Input: part model. Units: mm. Frame: model coordinates. A direction names the side the tool comes from. Coordinates: 2 decimals unless noted, no trailing zeros. Loops run counter-clockwise (first coordinate to the right, second up) from the corner with the lowest first, then second, coordinate; pieces in that order, holes last. Notation, with made-up numbers: (86.5, 65) - (111.5, 65) arc R9 cw to (111.5, 72) - close; hole circle Ø5 at (56, 72.25). An arc over 180 degrees is marked (long way). Use one line per item in the form item = value.
from build123d import *

# Parameters (mm, degrees)
CROQUIS1_W              = 93
CROQUIS1_H              = 56
SALIENTE_EXTRUIR1_DEPTH = 2.6
CROQUIS2_W              = 10
CROQUIS2_H              = 2.5
CORTAR_EXTRUIR1_DEPTH   = 2.6
CROQUIS3_W              = 6
CROQUIS3_H              = 1.5
CROQUIS3_H_2            = 3
SALIENTE_EXTRUIR2_DEPTH = 2.6


with BuildPart() as part:
    # Croquis1 → Saliente-Extruir1 (new body)
    with BuildSketch(Plane(origin=(0, 0, 0), x_dir=(1, 0, 0), z_dir=(0, 1, 0))):
        Rectangle(CROQUIS1_W, CROQUIS1_H)
    extrude(amount=SALIENTE_EXTRUIR1_DEPTH)

    # Croquis2 → Cortar-Extruir1 (cut)
    with BuildSketch(Plane(origin=(0, 2.6, 0), x_dir=(1, 0, 0), z_dir=(0, 1, 0))):
        with Locations((0, 26.75)):
            Rectangle(CROQUIS2_W, CROQUIS2_H)
    extrude(amount=-CORTAR_EXTRUIR1_DEPTH, mode=Mode.SUBTRACT)

    # Croquis3 → Saliente-Extruir2 (add)
    with BuildSketch(Plane.XZ):
        with Locations((13.5, 28.75)):
            Rectangle(CROQUIS3_W, CROQUIS3_H)
        with Locations((13.5, 26.5)):
            Rectangle(CROQUIS3_W, CROQUIS3_H_2)
        with Locations((-13.5, 28.75)):
            Rectangle(CROQUIS3_W, CROQUIS3_H)
        with Locations((-13.5, 26.5)):
            Rectangle(CROQUIS3_W, CROQUIS3_H_2)
    extrude(amount=SALIENTE_EXTRUIR2_DEPTH)


solid = part.part
Q1. Cut plane A-A, the plane x = -11.5. Return loops of the section in (y, z), then the cut area to 3 significant figures.
Check values:
outline = (-2.6, 25) - (0, 25) - (0, -28) - (2.6, -28) - (2.6, 28) - (0, 28) - (0, 29.5) - (-2.6, 29.5) - close
area = 157 mm²
Q2. Ray query, line 1 along Z through (x, y) = (-14, -0.9); line 2 along Z through (x, y) = (-27, 2.2); line 3 along Y through (x, z) = (-6, 14). Return the intervals inside material, ascending. Write a range as [from, to].
Check values:
line_1 = [25, 29.5]
line_2 = [-28, 28]
line_3 = [0, 2.6]
Q3. Pull-direction query (X, two-part tool) for faces 4 (the flat face through (-14, -1, 25)), 5 (the flat face through (-10.5, -1, 27)), 6 (the flat face through (-16.5, -1, 27)); classes: pulls with the +X half, pulls with the -X half, needs draft (parallel to the pull), parting line crosses it, or undercut.
Check values:
face_4 = needs draft
face_5 = undercut
face_6 = pulls with the -X half
Q4. Cut plane B-B, the plane z = 11.5. Return loops of the section in (x, y).
Check values:
outline = (-46.5, 0) - (46.5, 0) - (46.5, 2.6) - (-46.5, 2.6) - close
Q5. Cut plane C-C, the plane x = -36. Return loops of the section in (y, z), then the cut area to 3 significant figures.
Check values:
outline = (0, -28) - (2.6, -28) - (2.6, 28) - (0, 28) - close
area = 146 mm²
Q6. Set-up query: faces 1 (the flat face through (13, -1, 25)), 2 (the flat face through (0, 1, -25.5)), 3 (the flat face through (16.5, -1, 27)). Return all of +Z, -Z, +X, -X, +Y, -Y with unobstructed straight access to the full face (end or side cutting, diameter ignored); none if empty.
Check values:
face_1 = -Z, +X, -X, -Y
face_2 = -Z, +Y, -Y
face_3 = +Z, -Z, +X, -Y
Q7. First-contact query: P1, Ø0.8, axis at x = 7, y = 1, coming from the +Z side; P2, Ø0.8, axis at x = -13, z = 28.5, coming from the +Y side; P3, Ø1.3, axis at x = -1, y = 1, coming from the -Z side. Flat tips, straight axial feed; report the tip coordinate or a pass-through.
Check values:
P1 = 28
P2 = 0
P3 = -25.5
